```python
from build123d import *

# Parameters (mm, degrees)
SKETCH1_W            = 28
SKETCH1_H            = 3
BOSS_EXTRUDE1_DEPTH  = 7
SKETCH2_W            = 3
SKETCH2_H            = 7
BOSS_EXTRUDE2_DEPTH  = 26
SKETCH3_W            = 6
SKETCH3_H            = 7
BOSS_EXTRUDE3_DEPTH  = 27
BOSS_EXTRUDE4_DEPTH  = 7
CHAMFER1_SIZE        = 2
FILLET1_R            = 3
CUT_EXTRUDE1_DEPTH   = 8
SKETCH6_W            = 34
SKETCH6_H            = 7
BOSS_EXTRUDE5_DEPTH  = 25
SKETCH8_W            = 28
SKETCH8_H            = 21
CUT_EXTRUDE2_DEPTH   = 25
CHAMFER2_SIZE        = 3
FILLET2_R            = 1
SKETCH9_W            = 28
SKETCH9_H            = 4
BOSS_EXTRUDE6_DEPTH  = 7
SKETCH10_W           = 28
SKETCH10_H           = 2
BOSS_EXTRUDE7_DEPTH  = 4
CHAMFER3_SIZE        = 1
CHAMFER4_SIZE        = 3
CHAMFER5_SIZE        = 2
FILLET4_R            = 1.5
SKETCH11_W           = 14
SKETCH11_H           = 7
BOSS_EXTRUDE8_DEPTH  = 1
CHAMFER6_SIZE        = 1
SKETCH12_W           = 14
SKETCH12_H           = 7
BOSS_EXTRUDE9_DEPTH  = 1
CHAMFER7_SIZE        = 1
SKETCH13_W           = 30
SKETCH13_H           = 0.8
CUT_EXTRUDE3_DEPTH   = 12.7
SKETCH14_W           = 30
SKETCH14_H           = 0.8
CUT_EXTRUDE4_DEPTH   = 12.7
BOSS_EXTRUDE10_DEPTH = 5.4
FILLET5_R            = 5
CHAMFER8_SIZE        = 3
SKETCH16_W           = 28
SKETCH16_H           = 2
BOSS_EXTRUDE11_DEPTH = 2
CHAMFER9_SIZE        = 2
SKETCH17_W           = 30.68644474
SKETCH17_H           = 2
BOSS_EXTRUDE12_DEPTH = 2
CHAMFER10_SIZE       = 2
CHAMFER11_SIZE       = 1.5
CHAMFER12_SIZE       = 1


with BuildPart() as part:
    # Sketch1 → Boss-Extrude1 (new body)
    with BuildSketch(Plane(origin=(0, 0, 0), x_dir=(1, 0, 0), z_dir=(0, 1, 0))):
        Rectangle(SKETCH1_W, SKETCH1_H)
    extrude(amount=BOSS_EXTRUDE1_DEPTH)

    # Sketch2 → Boss-Extrude2 (add)
    with BuildSketch(Plane(origin=(0, 0, -1.5), x_dir=(-1, 0, 0), z_dir=(0, 0, -1))):
        with Locations((12.5, 3.5)):
            Rectangle(SKETCH2_W, SKETCH2_H)
        with Locations((-12.5, 3.5)):
            Rectangle(SKETCH2_W, SKETCH2_H)
    extrude(amount=BOSS_EXTRUDE2_DEPTH)

    # Sketch3 → Boss-Extrude3 (add)
    with BuildSketch(Plane(origin=(0, 0, -1.5), x_dir=(-1, 0, 0), z_dir=(0, 0, -1))):
        with Locations((0, 3.5)):
            Rectangle(SKETCH3_W, SKETCH3_H)
    extrude(amount=BOSS_EXTRUDE3_DEPTH)

    # Sketch4 → Boss-Extrude4 (add)
    with BuildSketch(Plane(origin=(0, 7, 0), x_dir=(1, 0, 0), z_dir=(0, 1, 0))):
        Polygon((-14, 12.5), (-15.7, 11.707276981), (-15.7, 16.707276981), (-14, 19.5), align=None)
        Polygon((14, 12.5), (15.7, 11.800538513), (15.7, 16.800538513), (14, 19.5), align=None)
    extrude(amount=-BOSS_EXTRUDE4_DEPTH)

    # Chamfer1
    chamfer1_edges = [part.edges().sort_by_distance(p)[0] for p in [
        (3, 3.5, -1.5),
        (-3, 3.5, -1.5),
    ]]
    chamfer(chamfer1_edges, length=CHAMFER1_SIZE)

    # Fillet1
    fillet1_edges = [part.edges().sort_by_distance(p)[0] for p in [
        (-11, 3.5, -1.5),
        (11, 3.5, -1.5),
    ]]
    fillet(fillet1_edges, radius=FILLET1_R)

    # Sketch5 → Cut-Extrude1 (cut)
    with BuildSketch(Plane(origin=(0, 7, 0), x_dir=(1, 0, 0), z_dir=(0, 1, 0))):
        Polygon((-14, 21.5), (-11, 27.5), (-14, 27.5), align=None)
        Polygon((14, 21.5), (11, 27.5), (14, 27.5), align=None)
    extrude(amount=-CUT_EXTRUDE1_DEPTH, mode=Mode.SUBTRACT)

    # Sketch6 → Boss-Extrude5 (add)
    with BuildSketch(Plane.XY.offset(1.5)):
        with Locations((0, 3.5)):
            Rectangle(SKETCH6_W, SKETCH6_H)
    extrude(amount=BOSS_EXTRUDE5_DEPTH)

    # Sketch8 → Cut-Extrude2 (cut)
    with BuildSketch(Plane(origin=(0, 7, 0), x_dir=(1, 0, 0), z_dir=(0, 1, 0))):
        with Locations((0, -14)):
            Rectangle(SKETCH8_W, SKETCH8_H)
    extrude(amount=-CUT_EXTRUDE2_DEPTH, mode=Mode.SUBTRACT)

    # Chamfer2
    chamfer2_edges = [part.edges().sort_by_distance(p)[0] for p in [
        (-14, 3.5, 3.5),
        (14, 3.5, 3.5),
    ]]
    chamfer(chamfer2_edges, length=CHAMFER2_SIZE)

    # Fillet2
    fillet2_edges = [part.edges().sort_by_distance(p)[0] for p in [
        (-17, 3.5, 1.5),
        (17, 3.5, 1.5),
    ]]
    fillet(fillet2_edges, radius=FILLET2_R)

    # Sketch9 → Boss-Extrude6 (add)
    with BuildSketch(Plane(origin=(0, 7, 0), x_dir=(1, 0, 0), z_dir=(0, 1, 0))):
        with Locations((0, -13.5)):
            Rectangle(SKETCH9_W, SKETCH9_H)
    extrude(amount=-BOSS_EXTRUDE6_DEPTH)

    # Sketch10 → Boss-Extrude7 (add)
    with BuildSketch(Plane(origin=(0, 0, 24.5), x_dir=(-1, 0, 0), z_dir=(0, 0, -1))):
        with Locations((0, 1)):
            Rectangle(SKETCH10_W, SKETCH10_H)
    extrude(amount=BOSS_EXTRUDE7_DEPTH)

    # Chamfer3
    chamfer3_edges = [part.edges().sort_by_distance(p)[0] for p in [
        (0, 2, 20.5),
    ]]
    chamfer(chamfer3_edges, length=CHAMFER3_SIZE)

    # Chamfer4
    chamfer4_edges = [part.edges().sort_by_distance(p)[0] for p in [
        (0, 2, 24.5),
    ]]
    chamfer(chamfer4_edges, length=CHAMFER4_SIZE - 0.0001)  # a hair under: the kernel refuses the full size

    # Chamfer5
    chamfer5_edges = [part.edges().sort_by_distance(p)[0] for p in [
        (0, 0, 15.5),
    ]]
    chamfer(chamfer5_edges, length=CHAMFER5_SIZE)

    # Fillet4
    fillet4_edges = [part.edges().sort_by_distance(p)[0] for p in [
        (3, 3.5, -28.5),
        (-3, 3.5, -28.5),
    ]]
    fillet(fillet4_edges, radius=FILLET4_R)

    # Sketch11 → Boss-Extrude8 (add)
    with BuildSketch(Plane(origin=(-11, 0, 0), x_dir=(0, 0, -1), z_dir=(1, 0, 0))):
        with Locations((20.5, 3.5)):
            Rectangle(SKETCH11_W, SKETCH11_H)
    extrude(amount=BOSS_EXTRUDE8_DEPTH)

    # Chamfer6
    chamfer6_edges = [part.edges().sort_by_distance(p)[0] for p in [
        (-10, 3.5, -13.5),
    ]]
    chamfer(chamfer6_edges, length=CHAMFER6_SIZE - 0.0001)  # a hair under: the kernel refuses the full size

    # Sketch12 → Boss-Extrude9 (add)
    with BuildSketch(Plane.ZY.offset(-11)):
        with Locations((-20.5, 3.5)):
            Rectangle(SKETCH12_W, SKETCH12_H)
    extrude(amount=BOSS_EXTRUDE9_DEPTH)

    # Chamfer7
    chamfer7_edges = [part.edges().sort_by_distance(p)[0] for p in [
        (10, 3.5, -13.5),
    ]]
    chamfer(chamfer7_edges, length=CHAMFER7_SIZE - 0.0001)  # a hair under: the kernel refuses the full size

    # Sketch13 → Cut-Extrude3 (cut)
    with BuildSketch(Plane(origin=(15.7, 0, 0), x_dir=(0, 0, -1), z_dir=(1, 0, 0))):
        with Locations((13.5, 6.6)):
            Rectangle(SKETCH13_W, SKETCH13_H)
        with Locations((13.5, 0.4)):
            Rectangle(SKETCH13_W, SKETCH13_H)
    extrude(amount=-CUT_EXTRUDE3_DEPTH, mode=Mode.SUBTRACT)

    # Sketch14 → Cut-Extrude4 (cut)
    with BuildSketch(Plane.ZY.offset(15.7)):
        with Locations((-13.5, 6.6)):
            Rectangle(SKETCH14_W, SKETCH14_H)
        with Locations((-13.5, 0.4)):
            Rectangle(SKETCH14_W, SKETCH14_H)
    extrude(amount=-CUT_EXTRUDE4_DEPTH, mode=Mode.SUBTRACT)

    # Sketch15 → Boss-Extrude10 (add)
    with BuildSketch(Plane(origin=(0, 6.2, 0), x_dir=(1, 0, 0), z_dir=(0, 1, 0))):
        Polygon((-15.7, 16.707276981), (-15.7, 20.746872846), (-11, 27.5), (-14, 19.5), align=None)
        Polygon((15.7, 16.800538513), (15.7, 20.746872846), (11, 27.5), (14, 19.5), align=None)
    extrude(amount=-BOSS_EXTRUDE10_DEPTH)

    # Fillet5
    fillet5_edges = [part.edges().sort_by_distance(p)[0] for p in [
        (-15.7, 3.5, -20.746872846),
        (15.7, 3.5, -20.746872846),
    ]]
    fillet(fillet5_edges, radius=FILLET5_R)

    # Chamfer8
    chamfer8_edges = [part.edges().sort_by_distance(p)[0] for p in [
        (0, 0, 26.5),
    ]]
    chamfer(chamfer8_edges, length=CHAMFER8_SIZE)

    # Sketch16 → Boss-Extrude11 (add)
    with BuildSketch(Plane(origin=(0, 0, 11.5), x_dir=(-1, 0, 0), z_dir=(0, 0, -1))):
        with Locations((0, 6)):
            Rectangle(SKETCH16_W, SKETCH16_H)
    extrude(amount=BOSS_EXTRUDE11_DEPTH)

    # Chamfer9
    chamfer9_edges = [part.edges().sort_by_distance(p)[0] for p in [
        (0, 5, 11.5),
    ]]
    chamfer(chamfer9_edges, length=CHAMFER9_SIZE - 0.0001)  # a hair under: the kernel refuses the full size

    # Sketch17 → Boss-Extrude12 (add)
    with BuildSketch(Plane.XY.offset(3.5)):
        with Locations((0.267537513, 1)):
            Rectangle(SKETCH17_W, SKETCH17_H)
    extrude(amount=BOSS_EXTRUDE12_DEPTH)

    # Chamfer10
    chamfer10_edges = [part.edges().sort_by_distance(p)[0] for p in [
        (0, 2, 3.5),
    ]]
    chamfer(chamfer10_edges, length=CHAMFER10_SIZE - 0.0001)  # a hair under: the kernel refuses the full size

    # Chamfer11
    chamfer11_edges = [part.edges().sort_by_distance(p)[0] for p in [
        (0, 7, 9.5),
    ]]
    chamfer(chamfer11_edges, length=CHAMFER11_SIZE)

    # Chamfer12
    chamfer12_edges = [part.edges().sort_by_distance(p)[0] for p in [
        (-14, 0.5, 20.5),
        (14, 0.5, 20.5),
    ]]
    chamfer(chamfer12_edges, length=CHAMFER12_SIZE - 0.0001)  # a hair under: the kernel refuses the full size


solid = part.part
```
Here's how the part is built. I have some questions about the finished solid (model axes, mm). A direction names the side the tool comes from. Coordinates: 2 decimals unless noted, no trailing zeros. Order: outer loops, then holes, each group sorted by start corner. A loop starts at its lowest first (then second) coordinate and runs counter-clockwise, first axis right, second up.
Item 1: If we section it at C-C, the plane z = -18: List the corners of the cut face in (x, y) for me.
Response values:
outline: (-15.7, 0.8) - (-10, 0.8) - (-10, 6.2) - (-15.7, 6.2) - close; (-3, 0) - (3, 0) - (3, 7) - (-3, 7) - close; (10, 0.8) - (15.7, 0.8) - (15.7, 6.2) - (10, 6.2) - close
Item 2: Which directions (+Z, -Z, +X, -X, +Y, -Y) give clear straight access to the entire face, cutting with the end or side of a thin tool? Please do faces 5 (the face through (0.2, 0.5, 20.5)), 6 (the face through (-10, 4, -21)), 7 (the face through (0.2, 4, 10.5)), 8 (the face through (0.2, 1.5, 21)).
Response values:
face 5: +Y, -Y
face 6: -Z, +Y, -Y
face 7: -Y
face 8: +Y
Item 3: If we section it at A-A, the plane z = -9: List the corners of the cut face in (x, y) for me, then the cut area to 3 significant figures.
Response values:
outline: (-14, 0.8) - (-11, 0.8) - (-11, 6.2) - (-14, 6.2) - close; (-3, 0) - (3, 0) - (3, 7) - (-3, 7) - close; (11, 0.8) - (14, 0.8) - (14, 6.2) - (11, 6.2) - close
area: 74.4 mm2
Item 4: If we section it at B-B, the plane x = 7: Give the number of separate pieces and of enclosed holes in the cut face, then the cut area to 3 significant figures.
Response values:
separate pieces: 3
enclosed holes: 0
area: 88.6 mm2
Item 5: I'm going to push flat-ended pins straight in: pin 1 Ø3.5 at (x, y) = (-9, 4.5) entering from -Z; pin 2 Ø1 at (x, y) = (-4, 6.5) entering from -Z; pin 3 Ø2.5 at (y, z) = (3.5, -18) entering from -X. Where does each tip first touch, or does it pass through?
Response values:
pin 1: stops at z = -27.5
pin 2: stops at z = -2.9
pin 3: stops at x = -15.7
Item 6: I need wall thicknesses on probe 1 along X at (y, z) = (5, -10.5); probe 2 along X at (y, z) = (2, -15.5); probe 3 along X at (y, z) = (5.5, 21.5). Which ranges of each line are inside material? Lowest first, please.
Response values:
probe 1: x = -14 to -11, -3 to 3, 11 to 14
probe 2: x = -15.7 to -10, -3 to 3, 10 to 15.7
probe 3: x = -17 to -14, 14 to 17
Item 7: Thinking about a two-plate mould opening in Z: for faces 1 (the face through (0, 6, 3.5)), 2 (the face through (-0.2, 3, 4.5)), 3 (the face through (-12.93, 3.54, -24.73)), 4 (the face through (-17, 3, 14)), which applies, pulls with the +Z half, pulls with the -Z half, needs draft (parallel to the pull), parting line crosses it, or undercut?
Response values:
face 1: undercut
face 2: undercut
face 3: pulls with the -Z half
face 4: needs draft
